```python
from build123d import *

# Parameters (mm, degrees)
EXTRUDE_1_DEPTH     = 2.5
CUT_EXTRUDE_1_DEPTH = 171.441338882
FILLET_1_R          = 10
FILLET_2_R          = 10
FILLET_3_R          = 10
FILLET_4_R          = 10
SKETCH_5_R          = 2.1
CUT_EXTRUDE_2_DEPTH = 171.441338882
SKETCH_6_R          = 1.5
CUT_EXTRUDE_3_DEPTH = 171.441338882
SKETCH_7_R          = 1.6
CUT_EXTRUDE_4_DEPTH = 171.441338882
CUT_EXTRUDE_5_DEPTH = 171.441338882
CUT_EXTRUDE_6_DEPTH = 171.441338882


with BuildPart() as part:
    # 草图1 → 凸台-拉伸1 (new body)
    with BuildSketch(Plane.XY):
        Polygon((-90, -35), (-90, -100), (90, -100), (90, -35), (138, -35), (138, 39), (90, 39), (90, 100), (-90, 100), (-90, 39), (-138, 39), (-138, -35), align=None)
    extrude(amount=EXTRUDE_1_DEPTH)

    # 草图4 → 切除-拉伸1 (cut, through all)
    with BuildSketch(Plane.XY.offset(2.5)):
        with BuildLine():
            Line((-45, 39.306212286), (-45, -30.693787714))
            ThreePointArc((-45, -30.693787714), (-50, -35.693787714), (-55, -30.693787714))
            Line((-55, -30.693787714), (-55, 39.306212286))
            ThreePointArc((-55, 39.306212286), (-50, 44.306212286), (-45, 39.306212286))
        make_face()
        with BuildLine():
            Line((5, 41.806212286), (5, -33.193787714))
            ThreePointArc((5, -33.193787714), (0, -38.193787714), (-5, -33.193787714))
            Line((-5, -33.193787714), (-5, 41.806212286))
            ThreePointArc((-5, 41.806212286), (0, 46.806212286), (5, 41.806212286))
        make_face()
        with BuildLine():
            Line((55, 39.306212286), (55, -30.693787714))
            ThreePointArc((55, -30.693787714), (50, -35.693787714), (45, -30.693787714))
            Line((45, -30.693787714), (45, 39.306212286))
            ThreePointArc((45, 39.306212286), (50, 44.306212286), (55, 39.306212286))
        make_face()
    extrude(amount=-CUT_EXTRUDE_1_DEPTH, mode=Mode.SUBTRACT)

    # 圆角1
    fillet_1_edges = [part.edges().sort_by_distance(p)[0] for p in [
        (-138, 39, 1.25),
    ]]
    fillet(fillet_1_edges, radius=FILLET_1_R)

    # 圆角2
    fillet_2_edges = [part.edges().sort_by_distance(p)[0] for p in [
        (-138, -35, 1.25),
    ]]
    fillet(fillet_2_edges, radius=FILLET_2_R)

    # 圆角3
    fillet_3_edges = [part.edges().sort_by_distance(p)[0] for p in [
        (138, -35, 1.25),
    ]]
    fillet(fillet_3_edges, radius=FILLET_3_R)

    # 圆角4
    fillet_4_edges = [part.edges().sort_by_distance(p)[0] for p in [
        (138, 39, 1.25),
    ]]
    fillet(fillet_4_edges, radius=FILLET_4_R)

    # 草图5 → 切除-拉伸2 (cut, through all)
    with BuildSketch(Plane(origin=(0, 0, 0), x_dir=(-1, 0, 0), z_dir=(0, 0, -1))):
        with Locations((-60, -89)):
            Circle(SKETCH_5_R)
        with Locations((-20, -89)):
            Circle(SKETCH_5_R)
        with Locations((20, -89)):
            Circle(SKETCH_5_R)
        with Locations((60, -89)):
            Circle(SKETCH_5_R)
    extrude(amount=-CUT_EXTRUDE_2_DEPTH, mode=Mode.SUBTRACT)

    # 草图6 → 切除-拉伸3 (cut, through all)
    with BuildSketch(Plane.XY.offset(2.5)):
        with Locations((-81, 90)):
            Circle(SKETCH_6_R)
        with Locations((-73, 90)):
            Circle(SKETCH_6_R)
        with Locations((-81, 62)):
            Circle(SKETCH_6_R)
        with Locations((-73, 62)):
            Circle(SKETCH_6_R)
        with Locations((73, 90)):
            Circle(SKETCH_6_R)
        with Locations((81, 90)):
            Circle(SKETCH_6_R)
        with Locations((73, 62)):
            Circle(SKETCH_6_R)
        with Locations((81, 62)):
            Circle(SKETCH_6_R)
        with Locations((-81, -58)):
            Circle(SKETCH_6_R)
        with Locations((-73, -58)):
            Circle(SKETCH_6_R)
        with Locations((-81, -86)):
            Circle(SKETCH_6_R)
        with Locations((-73, -86)):
            Circle(SKETCH_6_R)
        with Locations((73, -58)):
            Circle(SKETCH_6_R)
        with Locations((81, -58)):
            Circle(SKETCH_6_R)
        with Locations((73, -86)):
            Circle(SKETCH_6_R)
        with Locations((81, -86)):
            Circle(SKETCH_6_R)
    extrude(amount=-CUT_EXTRUDE_3_DEPTH, mode=Mode.SUBTRACT)

    # 草图7 → 切除-拉伸4 (cut, through all)
    with BuildSketch(Plane.XY.offset(2.5)):
        with Locations((-97, 29)):
            Circle(SKETCH_7_R)
        with Locations((-97, 2)):
            Circle(SKETCH_7_R)
        with Locations((-97, -25)):
            Circle(SKETCH_7_R)
        with Locations((97, 29)):
            Circle(SKETCH_7_R)
        with Locations((97, 2)):
            Circle(SKETCH_7_R)
        with Locations((97, -25)):
            Circle(SKETCH_7_R)
    extrude(amount=-CUT_EXTRUDE_4_DEPTH, mode=Mode.SUBTRACT)

    # 草图8 → 切除-拉伸5 (cut, through all)
    with BuildSketch(Plane.XY.offset(2.5)):
        with BuildLine():
            Line((-35, -61.3), (35, -61.3))
            ThreePointArc((35, -61.3), (36.6, -62.9), (35, -64.5))
            Line((35, -64.5), (-35, -64.5))
            ThreePointArc((-35, -64.5), (-36.6, -62.9), (-35, -61.3))
        make_face()
    extrude(amount=-CUT_EXTRUDE_5_DEPTH, mode=Mode.SUBTRACT)

    # 草图9 → 切除-拉伸6 (cut, through all)
    with BuildSketch(Plane.XY.offset(2.5)):
        with BuildLine():
            Line((65, 88.7), (-65, 88.7))
            ThreePointArc((-65, 88.7), (-66.6, 87.1), (-65, 85.5))
            Line((-65, 85.5), (65, 85.5))
            ThreePointArc((65, 85.5), (66.6, 87.1), (65, 88.7))
        make_face()
    extrude(amount=-CUT_EXTRUDE_6_DEPTH, mode=Mode.SUBTRACT)


solid = part.part
```
Geometry: final body of the model. Coordinates: model frame, mm. Round coordinates to 2 decimals unless told otherwise and drop trailing zeros.
Item 1: Line query: L1, parallel to Y at x = 6, z = 2.15; L2, parallel to X at y = 90, z = 1.2; L3, parallel to Y at x = -81, z = 0.5. Output: solid intervals per line, ascending.
Checked values:
L1: y = -100 to -64.5, -61.3 to 85.5, 88.7 to 100
L2: x = -90 to -82.5, -79.5 to -74.5, -71.5 to 71.5, 74.5 to 79.5, 82.5 to 90
L3: y = -100 to -87.5, -84.5 to -59.5, -56.5 to 60.5, 63.5 to 88.5, 91.5 to 100
Item 2: Contact query for flat-ended pins moving along their axis: P1, Ø0.8, axis at x = 102, z = 1, coming from the -Y side; P2, Ø2.5, axis at x = 60, y = -89, coming from the -Z side; P3, Ø0.8, axis at y = -79, z = 0.5, coming from the -X side. Output: stop coordinate, or through.
Checked values:
P1: stops at y = -35
P2: passes through
P3: stops at x = -90
Item 3: Section A-A, the plane z = 0.85. State how many separate pieces and enclosed holes the cut face has, plus the area to 3 significant figures.
Checked values:
separate pieces: 1
enclosed holes: 31
area: 39,800 mm2
